Could you check a few things on this drawing? It's one solid part, dimensions in mm from its lowest x, y, z. Coordinates: 2 decimals unless noted, no trailing zeros. Order: outer loops, then holes, each group sorted by start corner. A loop starts at its lowest first (then second) coordinate and runs counter-clockwise, first axis right, second up. Notation, with made-up numbers: (57.5, -2.5) -> (95.5, -2.5) arc R23 cw to (95.5, 32.5) -> close; hole circle Ø1 at (-19, -8.75). An arc over 180 degrees is marked (long way). Use a Markdown table: item, result. Add a question column.
1. Suppose I cut it at B-B, the plane x = 11. List the corners of the cut face in (y, z) for me (1 decimal), then the cut area to 3 significant figures.
2. If I drill on line 1 along Z through (x, y) = (23.95, 12.7); line 2 along X through (y, z) = (136, 39.5) (1 decimal); line 3 along Z through (x, y) = (4, 130.5) (1 decimal), over which ranges is the centre line in solid material (lowest first)? Write a range as from..to.
3. Suppose I cut it at A-A, the plane y = 355.6. List the corners of the cut face in (x, z) for me (1 decimal).
4. Suppose I cut it at D-D, the plane z = 7.5. List the corners of the cut face in (x, y) for me (1 decimal).
5. Suppose I cut it at C-C, the plane y = 168.5. List the corners of the cut face in (x, z) for me (1 decimal).
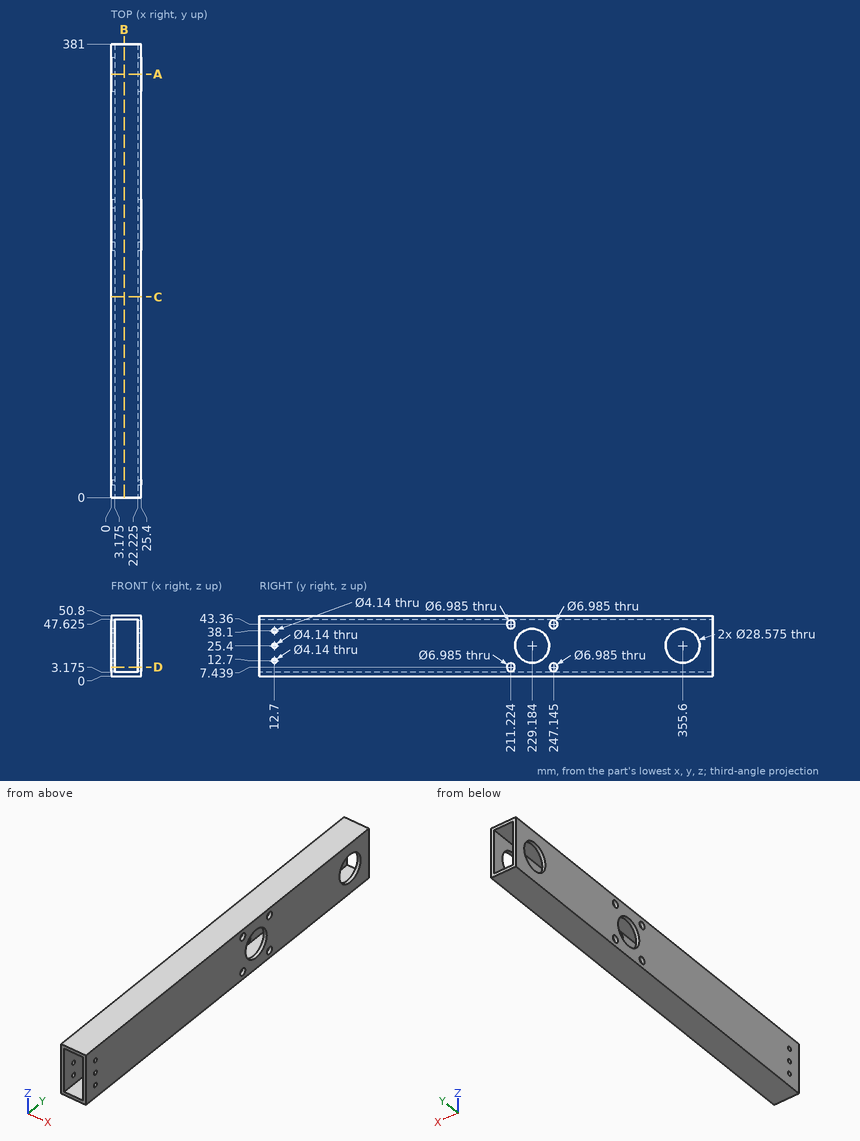
Worked out:
| question | item | result |
|---|---|---|
| 1 | outline | (0, 0) -> (381, 0) -> (381, 3.2) -> (0, 3.2) -> close; (0, 47.6) -> (381, 47.6) -> (381, 50.8) -> (0, 50.8) -> close |
| 1 | area | 2,420 mm² |
| 2 | line 1 | z = 0..10.63, 14.77..23.33, 27.47..36.03, 40.17..50.8 |
| 2 | line 2 | x = 0..3.2, 22.2..25.4 |
| 2 | line 3 | z = 0..3.2, 47.6..50.8 |
| 3 | outline | (0, 0) -> (25.4, 0) -> (25.4, 11.1) -> (22.2, 11.1) -> (22.2, 3.2) -> (3.2, 3.2) -> (3.2, 11.1) -> (0, 11.1) -> close; (0, 39.7) -> (3.2, 39.7) -> (3.2, 47.6) -> (22.2, 47.6) -> (22.2, 39.7) -> (25.4, 39.7) -> (25.4, 50.8) -> (0, 50.8) -> close |
| 4 | outline | (0, 0) -> (3.2, 0) -> (3.2, 207.7) -> (0, 207.7) -> close; (0, 214.7) -> (3.2, 214.7) -> (3.2, 243.7) -> (0, 243.7) -> close; (0, 250.6) -> (3.2, 250.6) -> (3.2, 381) -> (0, 381) -> close; (22.2, 0) -> (25.4, 0) -> (25.4, 207.7) -> (22.2, 207.7) -> close; (22.2, 214.7) -> (25.4, 214.7) -> (25.4, 243.7) -> (22.2, 243.7) -> close; (22.2, 250.6) -> (25.4, 250.6) -> (25.4, 381) -> (22.2, 381) -> close |
| 5 | outline | (0, 0) -> (25.4, 0) -> (25.4, 50.8) -> (0, 50.8) -> close; hole (3.2, 3.2) -> (22.2, 3.2) -> (22.2, 47.6) -> (3.2, 47.6) -> close |
